The listing builds one solid part. Answer for the finished solid, in the listing's coordinates (mm). A direction names the side the tool comes from. Coordinates: 2 decimals unless noted, no trailing zeros. Order: outer loops, then holes, each group sorted by start corner. A loop starts at its lowest first (then second) coordinate and runs counter-clockwise, first axis right, second up. Notation, with made-up numbers: (-39, 44) -> (-5, 44) arc R21 cw to (-5, 83) -> close; hole circle Ø5 at (41, 47). An arc over 180 degrees is marked (long way). Answer in a Markdown table with one row per item.
```python
from build123d import *

# Parameters (mm, degrees)
F0_W     = 745
F0_H     = 168
F1_DEPTH = 46
F3_DEPTH = 46
F4_W     = 42
F4_H     = 42
F5_DEPTH = 46


with BuildPart() as f1:
    # F0 (on Top) → F1 (new body)
    with BuildSketch(Plane.XY):
        with Locations((198.933674, -29.865599)):
            Rectangle(F0_W, F0_H)
    extrude(amount=F1_DEPTH)

    # F2 (on face) → F3 (cut)
    with BuildSketch(Plane.XY.offset(46)):
        Polygon((529.433674, -8.864585), (529.433674, -29.865599), (529.433674, -50.864585), (571.433674, -50.864585), (571.433674, -8.864585), align=None)
    extrude(amount=-F3_DEPTH, mode=Mode.SUBTRACT)

    # F4 (on face) → F5 (cut)
    with BuildSketch(Plane.XY.offset(46)):
        with Locations((-152.566326, -29.864585)):
            Rectangle(F4_W, F4_H)
    extrude(amount=-F5_DEPTH, mode=Mode.SUBTRACT)


solid = f1.part
```
(1) Flat-ended cylindrical pins translate along their axes: pin 1 (2 mm diameter, centred on y = -41.5, z = 35, fed in from -X); pin 2 (1 mm diameter, centred on y = -47.5, z = 36.5, fed in from +X). Find the tip coordinate at first contact, or state that the pin passes through.
Check values:
| item | result |
|---|---|
| pin 1 | x = -131.57 |
| pin 2 | x = 529.43 |
(2) Which of the six approach directions +Z, -Z, +X, -X, +Y, -Y give full straight-line access (tool end or side, diameter ignored) to faces 4 (the flat face through (194, 54.134, 23)), 5 (the flat face through (551, -8.865, 23)), 6 (the flat face through (-153, -8.865, 23))?
Check values:
| item | result |
|---|---|
| face 4 | +Z, -Z, +X, -X, +Y |
| face 5 | +Z, -Z, +X |
| face 6 | +Z, -Z, -X |
(3) A cutting plane is placed at A-A, the plane z = 33. Determine the outline of the cut face in (x, y).
Check values:
| item | result |
|---|---|
| outline | (-173.57, -113.87) -> (571.43, -113.87) -> (571.43, -50.86) -> (529.43, -50.86) -> (529.43, -8.86) -> (571.43, -8.86) -> (571.43, 54.13) -> (-173.57, 54.13) -> (-173.57, -8.86) -> (-131.57, -8.86) -> (-131.57, -50.86) -> (-173.57, -50.86) -> close |
(4) A cutting plane is placed at B-B, the plane y = -26. Determine the outline of the cut face in (x, z), then the cut area to 3 significant figures.
Check values:
| item | result |
|---|---|
| outline | (-131.57, 0) -> (529.43, 0) -> (529.43, 46) -> (-131.57, 46) -> close |
| area | 30,400 mm² |
(5) Find the intervals of material crossed by line 1 along X through (y, z) = (-30, 31.5), in increasing order. Write a range as from..to.
Check values:
| item | result |
|---|---|
| line 1 | -131.57..529.43 |
(6) For a pull along Y with two mould halves and no side action, classify faces 1 (the flat face through (194, -113.866, 23)), 2 (the flat face through (550, -50.865, 23)), 3 (the flat face through (571.434, 22, 23)) as released by +Y, released by -Y, zero draft, split by the parting line, or undercut.
Check values:
| item | result |
|---|---|
| face 1 | released by -Y |
| face 2 | undercut |
| face 3 | zero draft |
